Design review of the part built by this model. Coordinates are the model's own, in mm. A direction names the side the tool comes from. Coordinates: 2 decimals unless noted, no trailing zeros. Loops run counter-clockwise (first coordinate to the right, second up) from the corner with the lowest first, then second, coordinate; pieces in that order, holes last. Notation, with made-up numbers: (60, -12.5) - (83, -12.5) arc R27 cw to (83, 16.5) - close; hole circle Ø2 at (62, 88). An arc over 180 degrees is marked (long way). One line per question, with ' | ' between items.
from build123d import *

# Parameters (mm, degrees)
SKETCH2_W           = 40
SKETCH2_H           = 90
BOSS_EXTRUDE1_DEPTH = 5
SKETCH3_R           = 3.3
SKETCH3_R_2         = 9.7
CUT_EXTRUDE1_DEPTH  = 99.615414617
SKETCH5_R           = 1.7
CUT_EXTRUDE2_DEPTH  = 99.615414617


with BuildPart() as part:
    # Sketch2 → Boss-Extrude1 (new body)
    with BuildSketch(Plane(origin=(0, 0, 0), x_dir=(1, 0, 0), z_dir=(0, 1, 0))):
        with Locations((20, 45)):
            Rectangle(SKETCH2_W, SKETCH2_H)
    extrude(amount=BOSS_EXTRUDE1_DEPTH)

    # Sketch3 → Cut-Extrude1 (cut, through all)
    with BuildSketch(Plane(origin=(0, 5, 0), x_dir=(1, 0, 0), z_dir=(0, 1, 0))):
        with Locations(Location((20, 75.1, 0), (0, 0, 270))):
            Circle(SKETCH3_R)
        with Locations(Location((20, 45.1, 0), (0, 0, 270))):
            Circle(SKETCH3_R_2)
    extrude(amount=-CUT_EXTRUDE1_DEPTH, mode=Mode.SUBTRACT)

    # Sketch5 → Cut-Extrude2 (cut, through all)
    with BuildSketch(Plane(origin=(0, 5, 0), x_dir=(1, 0, 0), z_dir=(0, 1, 0))):
        with Locations(Location((11, 84.1, 0), (0, 0, 270))):
            Circle(SKETCH5_R)
        with Locations((11, 51.1)):
            Circle(SKETCH5_R)
    cut_extrude2 = extrude(amount=-CUT_EXTRUDE2_DEPTH, mode=Mode.SUBTRACT)

    # Mirror1: Cut-Extrude2 across plane
    add(cut_extrude2.mirror(Plane(origin=(20, 0, 0), x_dir=(0, 0, 1), z_dir=(1, 0, 0))), mode=Mode.SUBTRACT)


solid = part.part
Q1. For pin 1 (3 mm diameter, centred on x = 29, z = -51.1, fed in from -Y), flat-tipped, find the tip position at first contact; note if it passes through.
Returned:
pin 1: passes through
Q2. Take a section at D-D (z = -48). Give the boundary of the cut face in (x, y), plus the area to 3 significant figures.
Returned:
outline: (0, 0) - (10.74, 0) - (10.74, 5) - (0, 5) - close; (29.26, 0) - (40, 0) - (40, 5) - (29.26, 5) - close | area: 107 mm²
Q3. Take a section at C-C (y = 3.6). Give the boundary of the cut face in (x, z).
Returned:
outline: (0, -90) - (40, -90) - (40, 0) - (0, 0) - close; hole circle Ø3.4 at (11, -84.1); hole (11.32, -49.43) arc R1.7 ccw (long way) to (12.66, -51.45) arc R9.7 ccw to (27.34, -51.45) arc R1.7 ccw (long way) to (28.68, -49.43) arc R9.7 ccw (long way) to start; hole circle Ø6.6 at (20, -75.1); hole circle Ø3.4 at (29, -84.1)
Q4. Take a section at B-B (z = -84.1). Give the boundary of the cut face in (x, y), plus the area to 3 significant figures.
Returned:
outline: (0, 0) - (9.3, 0) - (9.3, 5) - (0, 5) - close; (12.7, 0) - (27.3, 0) - (27.3, 5) - (12.7, 5) - close; (30.7, 0) - (40, 0) - (40, 5) - (30.7, 5) - close | area: 166 mm²
Q5. Take a section at A-A (x = 20). Give the boundary of the cut face in (y, z).
Returned:
outline: (0, -90) - (5, -90) - (5, -78.4) - (0, -78.4) - close; (0, -71.8) - (5, -71.8) - (5, -54.8) - (0, -54.8) - close; (0, -35.4) - (5, -35.4) - (5, 0) - (0, 0) - close
Q6. To check wall thickness, follow line 1 along X through (y, z) = (3.3, -84.1); line 2 along Z through (x, y) = (17, 2); line 3 along X through (y, z) = (3.25, -75.1). State the ranges of each line that lie inside material, in increasing order.
Returned:
line 1: x = 0 to 9.3, 12.7 to 27.3, 30.7 to 40 | line 2: z = -90 to -76.47, -73.73 to -54.32, -35.88 to 0 | line 3: x = 0 to 16.7, 23.3 to 40
Q7. Tool access review of faces 1 (the cylindrical face through (20.1, 2.5, -54.8)), 2 (the flat face through (24, 0, -36)): name each direction out of +Z, -Z, +X, -X, +Y, -Y from which nothing blocks a thin tool from reaching the whole face with its end or side.
Returned:
face 1: +Y, -Y | face 2: +Z, -Z, +X, -X, -Y
Q8. Draft analysis for pull direction X (two halves, no side actions). For faces 3 (the flat face through (0, 2, -44)), 4 (the flat face through (24, 5, -36)), 5 (the cylindrical face through (30.38, 2.54, -52.09)), state which applies: +X half, -X half, draft (parallel to the pull), parting line (faces both ways), or undercut.
Returned:
face 3: -X half | face 4: draft | face 5: undercut
